Verification items for this drawing (mm, ordinates from the low corner). Give positions to 0.01 mm unless a question says otherwise; leave off trailing zeros. Loops run counter-clockwise (first coordinate to the right, second up) from the corner with the lowest first, then second, coordinate; pieces in that order, holes last. Notation, with made-up numbers: M 86,1.5 L 145,1.5 A14 ccw 145,26.5 Z; hole C -35.5,-32.5 d4. An arc over 180 degrees is marked long. Answer in a Markdown table with one row per item.
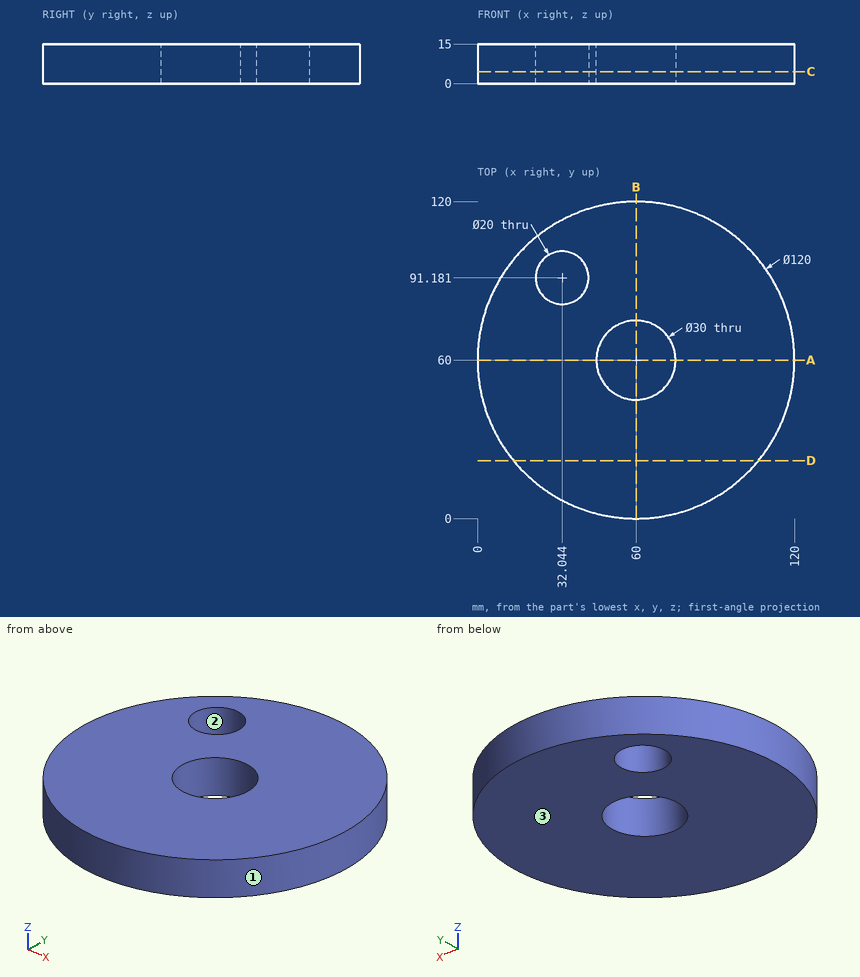
Item 1: Sectioned sample at D-D (y = 22). Record the cut outline in (x, z), and give its area (3 significant figures).
Reported:
| item | result |
|---|---|
| outline | M 13.57,0 L 106.43,0 L 106.43,15 L 13.57,15 Z |
| area | 1,390 mm^2 |
Item 2: Sectioned sample at A-A (y = 60). Record the cut outline in (x, z).
Reported:
| item | result |
|---|---|
| outline | M 0,0 L 45,0 L 45,15 L 0,15 Z; M 75,0 L 120,0 L 120,15 L 75,15 Z |
Item 3: Go/stop test with flat-tipped pins: pin 1 (6 mm diameter, centred on y = 97.5, z = 3, fed in from -X); pin 2 (18 mm diameter, centred on x = 60, y = 60, fed in from +Z); pin 3 (1.5 mm diameter, centred on x = 96, z = 3, fed in from +Y); pin 4 (4 mm diameter, centred on y = 17, z = 9.5, fed in from +X) (1 decimal). Record where each tip stops, or that it passes through.
Reported:
| item | result |
|---|---|
| pin 1 | stops at x = 10.91 |
| pin 2 | passes through |
| pin 3 | stops at y = 108.55 |
| pin 4 | stops at x = 103.8 |
Item 4: Scan lines: L1, parallel to Y at x = 60, z = 4; L2, parallel to Y at x = 29, z = 8.5 (1 decimal); L3, parallel to X at y = 50.5, z = 5.75 (1 decimal). Record each from-to range of solid material in increasing order. Write a range as [from, to].
Reported:
| item | result |
|---|---|
| L1 | y = [0, 45], [75, 120] |
| L2 | y = [8.6, 81.7], [100.7, 111.4] |
| L3 | x = [0.8, 48.4], [71.6, 119.2] |
Item 5: Release check for a two-part mould opening along X. For the marked faces 1, 2 and 3 record: released by +X, released by -X, zero draft, split by the parting line, or undercut.
Reported:
| item | result |
|---|---|
| face 1 | split by the parting line |
| face 2 | undercut |
| face 3 | zero draft |
Item 6: Sectioned sample at C-C (z = 4.5). Record the cut outline in (x, y) (1 decimal).
Reported:
| item | result |
|---|---|
| outline | C 60,60 d120; hole C 32,91.2 d20; hole C 60,60 d30 |
